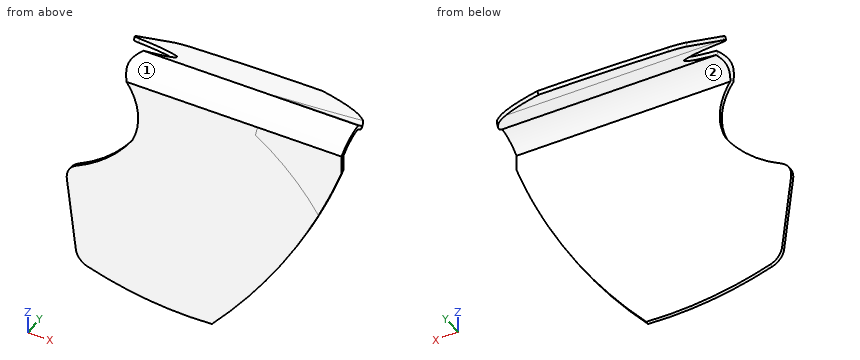
```python
from build123d import *

# Parameters (mm, degrees)
BOSS_EXTRUDE5_REACH            = 265.679
BOSS_EXTRUDE6_REACH            = 265.679
BOSS_EXTRUDE6_END_MAJOR_RADIUS = 41.29497886
BOSS_EXTRUDE6_END_MINOR_RADIUS = 34.238910582
CUT_EXTRUDE2_DEPTH             = 264.679090264
CUT_EXTRUDE2_DEPTH_BACK        = 264.679090264
SKETCH15_W                     = 51.852711212
SKETCH15_H                     = 208.671256167
CUT_EXTRUDE3_DEPTH             = 268.405797009
CUT_EXTRUDE3_TAPER             = -7
FILLET1_R                      = 10


with BuildPart() as part:
    # Sweep1: sweep along a path in Sketch9
    with BuildLine(Plane(origin=(0, 0, 0), x_dir=(0, 0, -1), z_dir=(1, 0, 0))) as sweep1_path:
        ThreePointArc((6.690833444, 0), (4.4769871, 9.372874687), (-1.696623298, 16.764655947))
    # Sketch3 → Sweep1 (sweep)
    with BuildSketch(Plane(origin=(0, 0, 0), x_dir=(1, 0, 0), z_dir=(0, 1, 0))):
        with BuildLine():
            Line((142.439103739, 11.914830112), (143.614236161, 6.690833444))
            Line((143.614236161, 6.690833444), (83.614236161, 6.690833444))
            Line((83.614236161, 6.690833444), (68.614236161, 6.690833444))
            ThreePointArc((68.614236161, 6.690833444), (75.180479735, 23.997298156), (71.779240838, 42.192375773))
            ThreePointArc((71.779240838, 42.192375773), (51.379079295, 63.12072091), (24.905577059, 75.502800726))
            ThreePointArc((24.905577059, 75.502800726), (11.315687886, 83.748123559), (5.247844857, 98.440016471))
            ThreePointArc((5.247844857, 98.440016471), (7.693142423, 109.618807389), (15.866887418, 117.62722417))
            ThreePointArc((15.866887418, 117.62722417), (96.637810578, 139.573762678), (179.070811064, 125.068832083))
            ThreePointArc((179.070811064, 125.068832083), (185.95529686, 120.311391566), (190.290589438, 113.153555076))
            Line((190.290589438, 113.153555076), (190.62158299, 112.199107439))
            ThreePointArc((190.62158299, 112.199107439), (191.44765289, 108.968802746), (191.725584387, 105.646151098))
            Line((191.725584387, 105.646151098), (191.725584387, 88.676044486))
            ThreePointArc((191.725584387, 88.676044486), (190.474138078, 74.473395816), (185.740302271, 61.024524277))
            ThreePointArc((185.740302271, 61.024524277), (167.286232208, 33.651220513), (142.439103739, 11.914830112))
        make_face()
    sweep(path=sweep1_path.line)

    # Boss-Extrude5: up to this cone (the profile starts outside it)
    boss_extrude5_end = Plane(origin=(191.725584, 0, 14.257299609), z_dir=(-1, 0, 0)).offset(43.399088878) * Cone(4.445e-06, 990.357764429, 222.779911122, align=(Align.CENTER, Align.CENTER, Align.MIN), mode=Mode.PRIVATE)
    # Sketch11 → Boss-Extrude5 (add, up to the surface)
    with BuildSketch(Plane(origin=(191.725584387, 0, 0), x_dir=(0, 0, -1), z_dir=(1, 0, 0)), mode=Mode.PRIVATE) as boss_extrude5_sk1:
        with BuildLine():
            Line((47.462397011, 82.376892243), (30.882313527, 60.247558735))
            Line((30.882313527, 60.247558735), (1.435728928, 20.945386831))
            ThreePointArc((1.435728928, 20.945386831), (9.148899919, 11.710260363), (11.914830112, 0))
            Line((11.914830112, 0), (61.024524277, 0))
            Line((61.024524277, 0), (88.676044486, 0))
            ThreePointArc((88.676044486, 0), (77.797814579, 46.055719281), (47.462397011, 82.376892243))
        make_face()
    boss_extrude5_tool1 = extrude(boss_extrude5_sk1.sketch, amount=-BOSS_EXTRUDE5_REACH, mode=Mode.PRIVATE) - boss_extrude5_end
    add(boss_extrude5_tool1.solids().sort_by_distance((191.725584, 31.140819, -47.986254))[0])

    # Boss-Extrude6: up to this torus (the profile starts outside it)
    boss_extrude6_end = Plane(origin=(41.076827722, 0, 14.257299609), z_dir=(1, 0, 0)) * Torus(BOSS_EXTRUDE6_END_MAJOR_RADIUS, BOSS_EXTRUDE6_END_MINOR_RADIUS, mode=Mode.PRIVATE)
    # Sketch12 → Boss-Extrude6 (add, up to the surface)
    with BuildSketch(Plane(origin=(191.725584387, 0, 0), x_dir=(0, 0, -1), z_dir=(1, 0, 0)), mode=Mode.PRIVATE) as boss_extrude6_sk1:
        with BuildLine():
            Line((1.435728928, 20.945386831), (-1.696623298, 16.764655947))
            ThreePointArc((-1.696623298, 16.764655947), (1.119891209, 7.693299714), (6.690833444, 0))
            Line((6.690833444, 0), (11.914830112, 0))
            ThreePointArc((11.914830112, 0), (9.148899919, 11.710260363), (1.435728928, 20.945386831))
        make_face()
    boss_extrude6_tool1 = extrude(boss_extrude6_sk1.sketch, amount=-BOSS_EXTRUDE6_REACH, mode=Mode.PRIVATE) - boss_extrude6_end
    add(boss_extrude6_tool1.solids().sort_by_distance((191.725584, 9.709782, -5.15039))[0])

    # Sketch14 → Cut-Extrude2 (cut, two sides: drawn at the far end of the back side and taken through both)
    with BuildSketch(Plane(origin=(191.725584387, 0, 0), x_dir=(0, 0, -1), z_dir=(1, 0, 0)).offset(-CUT_EXTRUDE2_DEPTH_BACK)):
        with BuildLine():
            Line((105.646151098, 2), (149.683498086, 2))
            Line((149.683498086, 2), (149.683498086, 144.664441597))
            Line((149.683498086, 144.664441597), (96.629526617, 144.664441597))
            Line((96.629526617, 144.664441597), (46.505246197, 77.763878679))
            Line((46.505246197, 77.763878679), (0.408030952, 16.238214412))
            ThreePointArc((0.408030952, 16.238214412), (2.90852666, 8.588164632), (7.531494019, 2))
            Line((7.531494019, 2), (84.410363787, 2))
            Line((84.410363787, 2), (88.676044486, 2))
            Line((88.676044486, 2), (105.646151098, 2))
        make_face()
    extrude(amount=CUT_EXTRUDE2_DEPTH + CUT_EXTRUDE2_DEPTH_BACK, mode=Mode.SUBTRACT)

    # Sketch15 → Cut-Extrude3 (cut, through all)
    with BuildSketch(Plane(origin=(0, 0, 0), x_dir=(1, 0, 0), z_dir=(0, -0.10182146993355343, 0.9948026881048173))):
        with Locations((-1.277666278, 17.910609482)):
            Rectangle(SKETCH15_W, SKETCH15_H)
    extrude(amount=-CUT_EXTRUDE3_DEPTH, taper=CUT_EXTRUDE3_TAPER, mode=Mode.SUBTRACT)

    # Fillet1
    fillet1_edges = [part.edges().sort_by_distance(p)[0] for p in [
        (40.347072898, 1.000004161, -128.41868422),
        (34.696815444, 111.874269162, -70.812250863),
        (30.333338635, 69.924766029, -39.382594446),
        (33.541632629, 1.000078518, -72.703242973),
    ]]
    fillet(fillet1_edges, radius=FILLET1_R)

    # Cut-Sweep1: sweep along a path in Sketch17
    with BuildLine(Plane(origin=(0, 0, 0), x_dir=(0, 0, -1), z_dir=(1, 0, 0))) as cut_sweep1_path:
        ThreePointArc((62.370921608, 102.275206583), (105.746248809, 53.324211599), (121.268282878, -10.210703039))
    # Sketch16 → Cut-Sweep1 (sweep, cut)
    with BuildSketch(Plane(origin=(0, 6.841546732, 9.131369543), x_dir=(1, 0, 0), z_dir=(0, 0.599608388931302, 0.8002935585916011))):
        with BuildLine():
            Line((95.683594782, 159.687794473), (195.090767436, 159.687794473))
            Line((195.090767436, 159.687794473), (195.090767436, 6.80339077))
            ThreePointArc((195.090767436, 6.80339077), (154.850931705, 89.399030557), (95.683594782, 159.687794473))
        make_face()
    sweep(path=cut_sweep1_path.line, mode=Mode.SUBTRACT)


solid = part.part
```
Here's how the part is built. I have some questions about the finished solid (model axes, mm). Face numbers are marked on the shaded views. Round coordinates to 2 decimals unless told otherwise and drop trailing zeros.
1. Will these pins go through, and if not, where does the flat tip stop? pin 1 (10 mm diameter, centred on x = 146.5, y = 26, fed in from +Z); pin 2 (8 mm diameter, centred on x = 75.5, z = -110, fed in from +Y).
Answers:
pin 1: stops at z = -1.48
pin 2: stops at y = 2
2. Thinking about a two-plate mould opening in Y: for the marked faces 1 and 2, which applies, released by +Y, released by -Y, zero draft, split by the parting line, or undercut?
Answers:
face 1: released by -Y
face 2: undercut
3. If I drill on probe 1 along Y at (x, z) = (128.5, -120); probe 2 along Y at (x, z) = (77, -39.5); probe 3 along Y at (x, z) = (137, -27), over which ranges is the centre line in solid material (lowest first)?
Answers:
probe 1: y = 0 to 2
probe 2: y = 0 to 2, 68.41 to 71.75
probe 3: y = 0 to 2, 51.73 to 55.07
